```python
from build123d import *

# Parameters (mm, degrees)
F1_DEPTH = 60
F2_DEPTH = 25
F3_DEPTH = 9


with BuildPart() as f1:
    # F0 (on Front) → F1 (new body, symmetric)
    with BuildSketch(Plane.XZ):
        Polygon((0, 20), (0, 0), (80, 0), (80, 20), (60, 20), align=None)
    extrude(amount=F1_DEPTH, both=True)

    # F0 (on Front) → F2 (join, symmetric)
    with BuildSketch(Plane.XZ):
        with BuildLine():
            Line((60, 20), (80, 20))
            Line((80, 20), (80, 35))
            ThreePointArc((80, 35), (84.393398, 45.606602), (95, 50))
            Line((95, 50), (100, 50))
            Line((100, 50), (125, 50))
            Line((125, 50), (125, 70))
            Line((125, 70), (100, 70))
            Line((100, 70), (95, 70))
            ThreePointArc((95, 70), (70.251263, 59.748737), (60, 35))
            Line((60, 35), (60, 20))
        make_face()
    extrude(amount=F2_DEPTH, both=True)

    # F0 (on Front) → F3 (join, symmetric)
    with BuildSketch(Plane.XZ):
        with BuildLine():
            ThreePointArc((95, 70), (41.322724, 56.736825), (0, 20))
            Line((0, 20), (60, 20))
            Line((60, 20), (60, 35))
            ThreePointArc((60, 35), (70.251263, 59.748737), (95, 70))
        make_face()
    extrude(amount=F3_DEPTH, both=True)

    # F0 (on Front) → F4 (revolve)
    with BuildSketch(Plane.XZ):
        Polygon((125, 75), (125, 70), (125, 50), (125, 45), (150, 45), (150, 75), align=None)
    revolve(axis=Axis((125, 0, 60), (0, 0, -1)))


solid = f1.part
```
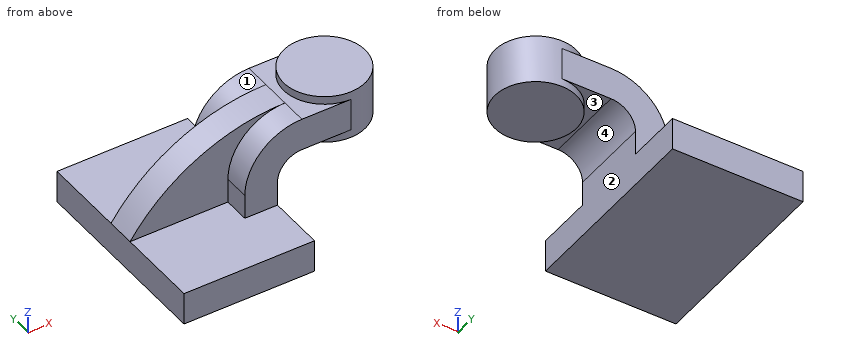
Geometry: final body of the model. Coordinates: model frame, mm. Face numbers are marked on the shaded views. A direction names the side the tool comes from. Round coordinates to 2 decimals unless told otherwise and drop trailing zeros. Order: outer loops, then holes, each group sorted by start corner. A loop starts at its lowest first (then second) coordinate and runs counter-clockwise, first axis right, second up. Notation, with made-up numbers: (-16.5, -39) -> (24.5, -39) arc R16 ccw to (24.5, -32) -> close; hole circle Ø4 at (55.5, 14.5). An arc over 180 degrees is marked (long way). Write each question's results on one line, items separated by ' | '.
Q1. Ray query, line 1 along X through (y, z) = (-28, 12); line 2 along Y through (x, z) = (117, 62); line 3 along Z through (x, y) = (98.5, 20). Return the intervals inside material, ascending.
Response values:
line 1: 0 to 80 | line 2: -25 to 25 | line 3: 50 to 70
Q2. Section query C-C (z = 8). Output: boundary loops of the cut face in (x, y), and give its area (3 significant figures).
Response values:
outline: (0, -60) -> (80, -60) -> (80, 60) -> (0, 60) -> close | area: 9,600 mm²
Q3. Pin query (flat end, axial travel): pin 1 Ø10.5 at (y, z) = (15, 13.5) entering from +X; pin 2 Ø7.5 at (y, z) = (19, 30.5) entering from -X; pin 3 Ø3 at (x, y) = (62, 19) entering from -Z; pin 4 Ø8 at (x, z) = (73, 34) entering from -Y. Return the tip coordinate at first contact, or that it passes through.
Response values:
pin 1: x = 80 | pin 2: x = 60 | pin 3: z = 0 | pin 4: y = -25
Q4. Access query for the marked faces 1, 2, 3 and 4. Directions: +Z, -Z, +X, -X, +Y, -Y. A direction counts if a zero-diameter tool reaches every point of the face in a straight line with its end or side. Return the directions, or none.
Response values:
face 1: +Z, -X, +Y | face 2: -Z, +X, +Y, -Y | face 3: -Z | face 4: -Z, +Y, -Y
Q5. Section query A-A (y = 20). Output: boundary loops of the cut face in (x, z), and give its area (3 significant figures).
Response values:
outline: (0, 0) -> (80, 0) -> (80, 35) arc R15 cw to (95, 50) -> (110, 50) -> (110, 45) -> (140, 45) -> (140, 75) -> (110, 75) -> (110, 70) -> (95, 70) arc R35 ccw to (60, 35) -> (60, 20) -> (0, 20) -> close | area: 3,890 mm²
Q6. Section query D-D (y = 0). Output: boundary loops of the cut face in (x, z), and give its area (3 significant figures).
Response values:
outline: (0, 0) -> (80, 0) -> (80, 35) arc R15 cw to (95, 50) -> (100, 50) -> (100, 45) -> (150, 45) -> (150, 75) -> (100, 75) -> (100, 70) -> (95, 70) arc R115.25 ccw to (0, 20) -> close | area: 6,130 mm²
Q7. Section query B-B (x = 25). Output: boundary loops of the cut face in (y, z), and give its area (3 significant figures).
Response values:
outline: (-60, 0) -> (60, 0) -> (60, 20) -> (9, 20) -> (9, 46.31) -> (-9, 46.31) -> (-9, 20) -> (-60, 20) -> close | area: 2,870 mm²
